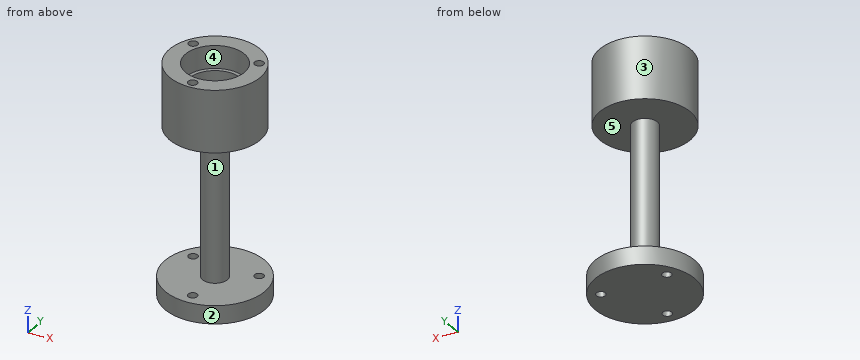
```python
from build123d import *

# Parameters (mm, degrees)
MOUNTING_FLANGE_START                          = -4
SKETCH1_R                                      = 11
MOUNTING_FLANGE_DEPTH                          = 4
SKETCH2_R                                      = 2.75
D5P5_CENTRAL_POST_DEPTH                        = 32.81
CLOSED_FLOOR_BELOW_SHAFT_NOSE_START            = 32.8
SKETCH3_R                                      = 10
CLOSED_FLOOR_BELOW_SHAFT_NOSE_DEPTH            = 2.2
SHAFT_AND_CLIP_CLEARANCE_START                 = 35
SKETCH4_R                                      = 10
SKETCH4_R_2                                    = 5.7
SHAFT_AND_CLIP_CLEARANCE_DEPTH                 = 6.5
LOWER_686ZZ_SEAT_START                         = 41.5
SKETCH5_R                                      = 10
SKETCH5_R_2                                    = 6.5
LOWER_686ZZ_SEAT_DEPTH                         = 5
SKETCH6_R                                      = 1
BASE_THREE_M2_THROUGH_THREAD_MAJOR_ENVEL_DEPTH = 4.01
TOP_CAP_THREE_M2_BLIND_THREAD_MAJOR_ENVE_START = -4.3
SKETCH7_R                                      = 1
TOP_CAP_THREE_M2_BLIND_THREAD_MAJOR_ENVE_DEPTH = 4.3


with BuildPart() as part:
    # Sketch1 → Mounting_Flange (new body)
    with BuildSketch(Plane.XY.offset(MOUNTING_FLANGE_START)):
        Circle(SKETCH1_R)
    extrude(amount=MOUNTING_FLANGE_DEPTH)

    # Sketch2 → D5p5_Central_Post (add)
    with BuildSketch(Plane.XY):
        Circle(SKETCH2_R)
    extrude(amount=D5P5_CENTRAL_POST_DEPTH)

    # Sketch3 → Closed_Floor_Below_Shaft_Nose (add)
    with BuildSketch(Plane.XY.offset(CLOSED_FLOOR_BELOW_SHAFT_NOSE_START)):
        Circle(SKETCH3_R)
    extrude(amount=CLOSED_FLOOR_BELOW_SHAFT_NOSE_DEPTH)

    # Sketch4 → Shaft_And_Clip_Clearance (add)
    with BuildSketch(Plane.XY.offset(SHAFT_AND_CLIP_CLEARANCE_START)):
        Circle(SKETCH4_R)
        with Locations(Location((0, 0, 0), (0, 0, 180))):
            Circle(SKETCH4_R_2, mode=Mode.SUBTRACT)
    extrude(amount=SHAFT_AND_CLIP_CLEARANCE_DEPTH)

    # Sketch5 → Lower_686ZZ_Seat (add)
    with BuildSketch(Plane.XY.offset(LOWER_686ZZ_SEAT_START)):
        Circle(SKETCH5_R)
        Circle(SKETCH5_R_2, mode=Mode.SUBTRACT)
    extrude(amount=LOWER_686ZZ_SEAT_DEPTH)

    # Sketch6 → Base_Three_M2_Through_Thread_Major_Envelopes (cut)
    with BuildSketch(Plane(origin=(0, 0, -4), x_dir=(-1, 0, 0), z_dir=(0, 0, -1))):
        with Locations((-7.188010851, 4.15)):
            Circle(SKETCH6_R)
        with Locations((7.188010851, 4.15)):
            Circle(SKETCH6_R)
        with Locations((0, -8.3)):
            Circle(SKETCH6_R)
    extrude(amount=-BASE_THREE_M2_THROUGH_THREAD_MAJOR_ENVEL_DEPTH, mode=Mode.SUBTRACT)

    # Sketch7 → Top_Cap_Three_M2_Blind_Thread_Major_Envelopes (cut)
    with BuildSketch(Plane.XY.offset(46.5).offset(TOP_CAP_THREE_M2_BLIND_THREAD_MAJOR_ENVE_START)):
        with Locations(Location((7.188010851, 4.15, 0), (0, 0, 180))):
            Circle(SKETCH7_R)
        with Locations(Location((-7.188010851, 4.15, 0), (0, 0, 180))):
            Circle(SKETCH7_R)
        with Locations(Location((0, -8.3, 0), (0, 0, 180))):
            Circle(SKETCH7_R)
    extrude(amount=TOP_CAP_THREE_M2_BLIND_THREAD_MAJOR_ENVE_DEPTH, mode=Mode.SUBTRACT)


solid = part.part
```
Input: part model. Units: mm. Frame: model coordinates. Face numbers are marked on the shaded views. A direction names the side the tool comes from. Round coordinates to 2 decimals unless told otherwise and drop trailing zeros. Loops run counter-clockwise (first coordinate to the right, second up) from the corner with the lowest first, then second, coordinate; pieces in that order, holes last. Notation, with made-up numbers: M 49,30.25 L 63,30.25 A21 cw 63,58.25 Z; hole C 63.25,85.25 d7. An arc over 180 degrees is marked long. Answer in a Markdown table with one row per item. Add a question column.
1. Section D-D (y = -8.3). Output: boundary loops of the cut face in (x, z).
2. Ray query, probe 1 along Y at (x, z) = (0, 43.7); probe 2 along Y at (x, z) = (0, -0.85); probe 3 along Z at (x, y) = (0, 4.5). Return the intervals inside material, ascending.
3. Contact query for flat-ended pins moving along their axis: pin 1 (6 mm diameter, centred on y = 6, z = 34.5, fed in from +X); pin 2 (1.5 mm diameter, centred on x = -3, z = 21.5, fed in from -Y); pin 3 (8 mm diameter, centred on x = -3, z = 23.5, fed in from +Y); pin 4 (1 mm diameter, centred on x = -5, z = 30, fed in from +Y). Output: stop coordinate, or through.
4. Set-up query: the marked faces 1 and 2. Return all of +Z, -Z, +X, -X, +Y, -Y with unobstructed straight access to the full face (end or side cutting, diameter ignored); none if empty.
5. Mould query, pull axis Y, two halves, no side actions, for the marked faces 3, 4 and 5. Classes: released by +Y, released by -Y, zero draft, split by the parting line, or undercut.
6. Section C-C (y = 7). Output: boundary loops of the cut face in (x, z).
7. Section B-B (y = 0). Output: boundary loops of the cut face in (x, z).
8. Section A-A (x = 0). Output: boundary loops of the cut face in (y, z).
Values follow:
| question | item | result |
|---|---|---|
| 1 | outline | M -7.22,-4 L -1,-4 L -1,0 L -7.22,0 Z; M -5.58,32.8 L 5.58,32.8 L 5.58,46.5 L 1,46.5 L 1,42.2 L -1,42.2 L -1,46.5 L -5.58,46.5 Z; M 1,-4 L 7.22,-4 L 7.22,0 L 1,0 Z |
| 2 | probe 1 | -10 to -9.3, -7.3 to -6.5, 6.5 to 10 |
| 2 | probe 2 | -11 to -9.3, -7.3 to 11 |
| 2 | probe 3 | -4 to 0, 32.8 to 35 |
| 3 | pin 1 | x = 9.54 |
| 3 | pin 2 | y = -1.58 |
| 3 | pin 3 | y = 2.75 |
| 3 | pin 4 | through |
| 4 | face 1 | none |
| 4 | face 2 | +Z, -Z |
| 5 | face 3 | split by the parting line |
| 5 | face 4 | undercut |
| 5 | face 5 | zero draft |
| 6 | outline | M -8.49,-4 L 8.49,-4 L 8.49,0 L -8.49,0 Z; M -7.14,32.8 L 7.14,32.8 L 7.14,46.5 L -7.14,46.5 Z |
| 7 | outline | M -11,-4 L 11,-4 L 11,0 L 2.75,0 L 2.75,32.8 L 10,32.8 L 10,46.5 L 6.5,46.5 L 6.5,41.5 L 5.7,41.5 L 5.7,35 L -5.7,35 L -5.7,41.5 L -6.5,41.5 L -6.5,46.5 L -10,46.5 L -10,32.8 L -2.75,32.8 L -2.75,0 L -11,0 Z |
| 8 | outline | M -11,-4 L -9.3,-4 L -9.3,0 L -11,0 Z; M -10,32.8 L -2.75,32.8 L -2.75,0 L -7.3,0 L -7.3,-4 L 11,-4 L 11,0 L 2.75,0 L 2.75,32.8 L 10,32.8 L 10,46.5 L 6.5,46.5 L 6.5,41.5 L 5.7,41.5 L 5.7,35 L -5.7,35 L -5.7,41.5 L -6.5,41.5 L -6.5,46.5 L -7.3,46.5 L -7.3,42.2 L -9.3,42.2 L -9.3,46.5 L -10,46.5 Z |
